For this review, use the dimensioned drawing (mm, ordinates from the lowest corner) and the shaded views. Coordinates: 2 decimals unless noted, no trailing zeros. Loops run counter-clockwise (first coordinate to the right, second up) from the corner with the lowest first, then second, coordinate; pieces in that order, holes last. Notation, with made-up numbers: (-23, 76.25) - (-4, 76.25) arc R11 ccw to (-4, 92.25) - close; hole circle Ø10 at (-37, -20.75). An arc over 180 degrees is marked (long way). Return JSON: item names as keys, results as strings. Group by question number.
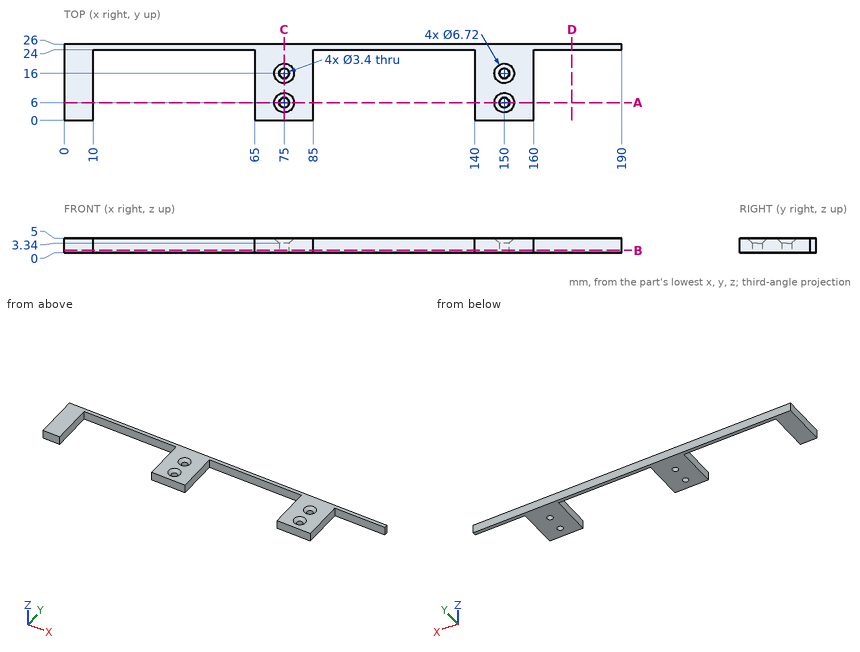
Item 1: Add section D-D (x = 173). State the section outline as (y, z) points, then the cut area to 3 significant figures.
Item 2: For P1, Ø12, axis at x = 112.5, y = 19, coming from the +Z side; P2, Ø4.5, axis at x = 75, y = 6, coming from the +Z side; P3, Ø2.5, axis at y = 8.5, z = 2, coming from the +X side; P4, Ø2.5, axis at x = 105.5, z = 1.5, coming from the -Y side, all flat-tipped, find the tip position at first contact; note any pin that passes through.
Item 3: To check wall thickness, follow line 1 (X direction, y = 6, z = 2.55); line 2 (Y direction, x = 75, z = 0.85); line 3 (X direction, y = 3, z = 2.35). State the ranges of each line that lie inside material, in increasing order. Write a range as from..to.
Item 4: Add section C-C (x = 75). State the section outline as (y, z) points.
Item 5: Add section A-A (y = 6). State the section outline as (x, z) points.
Item 6: Add section B-B (z = 0.85). State the section outline as (x, y) points.
Answers below:
{
 "1": {"outline": "(24, 0) - (26, 0) - (26, 5) - (24, 5) - close", "area": "10.0 mm^2"},
 "2": {"P1": "stops at z = 5", "P2": "stops at z = 3.89", "P3": "stops at x = 160", "P4": "stops at y = 24"},
 "3": {"line 1": "x = 0..10, 65..73.3, 76.7..85, 140..148.3, 151.7..160", "line 2": "y = 0..4.3, 7.7..14.3, 17.7..26", "line 3": "x = 0..10, 65..85, 140..160"},
 "4": {"outline": "(0, 0) - (4.3, 0) - (4.3, 3.34) - (2.64, 5) - (0, 5) - close; (7.7, 0) - (14.3, 0) - (14.3, 3.34) - (12.64, 5) - (9.36, 5) - (7.7, 3.34) - close; (17.7, 0) - (26, 0) - (26, 5) - (19.36, 5) - (17.7, 3.34) - close"},
 "5": {"outline": "(0, 0) - (10, 0) - (10, 5) - (0, 5) - close; (65, 0) - (73.3, 0) - (73.3, 3.34) - (71.64, 5) - (65, 5) - close; (76.7, 0) - (85, 0) - (85, 5) - (78.36, 5) - (76.7, 3.34) - close; (140, 0) - (148.3, 0) - (148.3, 3.34) - (146.64, 5) - (140, 5) - close; (151.7, 0) - (160, 0) - (160, 5) - (153.36, 5) - (151.7, 3.34) - close"},
 "6": {"outline": "(0, 0) - (10, 0) - (10, 24) - (65, 24) - (65, 0) - (85, 0) - (85, 24) - (140, 24) - (140, 0) - (160, 0) - (160, 24) - (190, 24) - (190, 26) - (0, 26) - close; hole circle Ø3.4 at (75, 6); hole circle Ø3.4 at (75, 16); hole circle Ø3.4 at (150, 6); hole circle Ø3.4 at (150, 16)"}
}
